```python
from build123d import *

# Parameters (mm, degrees)
SKETCH1_W           = 77.2
SKETCH1_H           = 20
SKETCH1_W_2         = 16
SKETCH1_H_2         = 16
BOSS_EXTRUDE1_DEPTH = 14
SKETCH2_W           = 77.2
SKETCH2_H           = 20
BOSS_EXTRUDE2_DEPTH = 2


with BuildPart() as part:
    # Sketch1 → Boss-Extrude1 (new body)
    with BuildSketch(Plane(origin=(0, 0, 0), x_dir=(1, 0, 0), z_dir=(0, 1, 0))):
        Rectangle(SKETCH1_W, SKETCH1_H)
        with Locations((-9.6, 0)):
            Rectangle(SKETCH1_W_2, SKETCH1_H_2, mode=Mode.SUBTRACT)
        with Locations((-28.6, 0)):
            Rectangle(SKETCH1_W_2, SKETCH1_H_2, mode=Mode.SUBTRACT)
        with Locations((9.4, 0)):
            Rectangle(SKETCH1_W_2, SKETCH1_H_2, mode=Mode.SUBTRACT)
        with Locations((28.4, 0)):
            Rectangle(SKETCH1_W_2, SKETCH1_H_2, mode=Mode.SUBTRACT)
    extrude(amount=BOSS_EXTRUDE1_DEPTH)

    # Sketch2 → Boss-Extrude2 (add)
    with BuildSketch(Plane(origin=(0, 14, 0), x_dir=(1, 0, 0), z_dir=(0, 1, 0))):
        Rectangle(SKETCH2_W, SKETCH2_H)
    extrude(amount=BOSS_EXTRUDE2_DEPTH)


solid = part.part
```
Model file for the job. Use its own axes, mm. A direction names the side the tool comes from. Coordinates: 2 decimals unless noted, no trailing zeros. Order: outer loops, then holes, each group sorted by start corner. A loop starts at its lowest first (then second) coordinate and runs counter-clockwise, first axis right, second up. Notation, with made-up numbers: (53.5, 17) -> (75.5, 17) arc R7 ccw to (75.5, 26) -> close; hole circle Ø3 at (77.5, 63.25). An arc over 180 degrees is marked (long way). Answer as a JSON object with one key per item and string values. Group by question number.
1) Pull direction Z, two halves, no side cores. Call faces 3 (the face through (-29, 14, 0)), 4 (the face through (-1, 8, -10)), 5 (the face through (-38.6, 8, 0)), 6 (the face through (-17.6, 7, 0)): +Z half, -Z half, draft (parallel to the pull), parting line (faces both ways), or undercut.
2) Drill centre lines: L1, parallel to X at y = 5, z = -7.5; L2, parallel to Z at x = 9.5, y = 10.75; L3, parallel to Y at x = 21, z = -7.25. Where is each one in solid material? Low to high.
3) Which spindle directions (+Z, -Z, +X, -X, +Y, -Y) get a long thin tool onto all of the face, cutting with end or side? Do faces 1 (the face through (-20.6, 7, 0)), 2 (the face through (-1, 16, 0)). Say none if no direction does.
4) Flat gauge pin, fed straight in: pin 1 (8 mm diameter, centred on x = -30, z = 1, fed in from -Y). Where does the tip first touch, or does it go through?
5) Cut at B-B, the plane z = -1.25. Write the cut outline in (x, y).
6) Cut at A-A, the plane y = 8.25. Write the cut outline in (x, z), then the cut area to 3 significant figures.
7) Cut at C-C, the plane x = -21.5. Write the cut outline in (y, z), then the cut area to 3 significant figures.
Check values:
{
 "1": {"face 3": "undercut", "face 4": "-Z half", "face 5": "draft", "face 6": "undercut"},
 "2": {"L1": "x = -38.6 to -36.6, -20.6 to -17.6, -1.6 to 1.4, 17.4 to 20.4, 36.4 to 38.6", "L2": "z = -10 to -8, 8 to 10", "L3": "y = 14 to 16"},
 "3": {"face 1": "-Y", "face 2": "+Z, -Z, +X, -X, +Y"},
 "4": {"pin 1": "stops at y = 14"},
 "5": {"outline": "(-38.6, 0) -> (-36.6, 0) -> (-36.6, 14) -> (-20.6, 14) -> (-20.6, 0) -> (-17.6, 0) -> (-17.6, 14) -> (-1.6, 14) -> (-1.6, 0) -> (1.4, 0) -> (1.4, 14) -> (17.4, 14) -> (17.4, 0) -> (20.4, 0) -> (20.4, 14) -> (36.4, 14) -> (36.4, 0) -> (38.6, 0) -> (38.6, 16) -> (-38.6, 16) -> close"},
 "6": {"outline": "(-38.6, -10) -> (38.6, -10) -> (38.6, 10) -> (-38.6, 10) -> close; hole (-36.6, -8) -> (-20.6, -8) -> (-20.6, 8) -> (-36.6, 8) -> close; hole (-17.6, -8) -> (-1.6, -8) -> (-1.6, 8) -> (-17.6, 8) -> close; hole (1.4, -8) -> (17.4, -8) -> (17.4, 8) -> (1.4, 8) -> close; hole (20.4, -8) -> (36.4, -8) -> (36.4, 8) -> (20.4, 8) -> close", "area": "520 mm²"},
 "7": {"outline": "(0, -10) -> (16, -10) -> (16, 10) -> (0, 10) -> (0, 8) -> (14, 8) -> (14, -8) -> (0, -8) -> close", "area": "96.0 mm²"}
}
